Part model, mm, in its own coordinate system. Give positions to 0.01 mm unless a question says otherwise; leave off trailing zeros. Write each loop counter-clockwise with the first axis right and the second up, starting at its lowest first coordinate (ties: lowest second). Pieces come first, ordered by that corner, then holes. Notation, with made-up numbers: (48, 65.5) - (102, 65.5) arc R19 cw to (102, 69.5) - close; hole circle Ø10 at (76.5, 8). An arc over 180 degrees is marked (long way). Answer in a Markdown table with one row per item. Add a question column.
1. Probe line 1 along X through (y, z) = (3.5, -6.5); line 2 along X through (y, z) = (4.75, -0.25); line 3 along X through (y, z) = (6.75, 4). List the from-to ranges inside material, lowest first.
2. Band-saw the part on A-A on y = 6.5. Write the cut outline in (x, z), plus the area to 3 significant figures.
3. Drop flat-ended pins along their axis: pin 1 Ø2 at (y, z) = (7, 6) entering from -X; pin 2 Ø11 at (x, z) = (0, 0) entering from -Y; pin 3 Ø2 at (y, z) = (5.5, 2.5) entering from -X. Give the stop position or say it passes through.
4. Pull direction Z, two halves, no side cores. Call faces 1 (the conical face through (-6.77, 7.72, 11.66)), 2 (the flat face through (-11.2, 3.9, -6.6)), 3 (the cylindrical face through (1.802, 4.056, 5.723)): released by +Z, released by -Z, zero draft, split by the parting line, or undercut.
5. Band-saw the part on B-B on y = 0.5. Write the cut outline in (x, z).
```python
from build123d import *

# Parameters (mm, degrees)
BOSS_EXTRUDE1_DEPTH     = 8
SKETCH2_R               = 6
CUT_EXTRUDE1_DEPTH      = 22.408720964
SKETCH3_OUTSIDE_W       = 67.838
SKETCH3_OUTSIDE_H       = 63.816
SKETCH3_OUTSIDE_R       = 13
CUT_EXTRUDE2_DEPTH      = 8
CUT_EXTRUDE2_DRAFT      = -60
MIRROR1_COPY_1_SKETCH_W = 67.838
MIRROR1_COPY_1_SKETCH_H = 63.816
MIRROR1_COPY_1_SKETCH_R = 13
MIRROR1_COPY_1_DEPTH    = 8
MIRROR1_COPY_1_DRAFT    = -60


with BuildPart() as part:
    # Sketch1 → Boss-Extrude1 (new body)
    with BuildSketch(Plane(origin=(0, 0, 0), x_dir=(1, 0, 0), z_dir=(0, 1, 0))):
        Polygon((7.505553499, -13), (15.011106999, 0), (7.505553499, 13), (-7.505553499, 13), (-15.011106999, 0), (-7.505553499, -13), align=None)
    extrude(amount=BOSS_EXTRUDE1_DEPTH)

    # Sketch2 → Cut-Extrude1 (cut, through all)
    with BuildSketch(Plane(origin=(0, 8, 0), x_dir=(1, 0, 0), z_dir=(0, 1, 0))):
        with Locations(Location((0, 0, 0), (0, 0, 270))):
            Circle(SKETCH2_R)
    extrude(amount=-CUT_EXTRUDE1_DEPTH, mode=Mode.SUBTRACT)


with BuildPart() as cut_extrude2_tool:
    # Sketch3 outside → Cut-Extrude2 (with draft: the straight prism first)
    with BuildSketch(Plane(origin=(0, 8, 0), x_dir=(1, 0, 0), z_dir=(0, 1, 0))):
        Rectangle(SKETCH3_OUTSIDE_W, SKETCH3_OUTSIDE_H)
        Circle(SKETCH3_OUTSIDE_R, mode=Mode.SUBTRACT)
    extrude(amount=-CUT_EXTRUDE2_DEPTH)
    # Cut-Extrude2: the draft: its side faces are tilted about the plane it starts from
    cut_extrude2_sides = [cut_extrude2_tool.faces().sort_by_distance(p)[0] for p in [
        (0, 4, 31.908),
        (33.919, 4, 0),
        (0, 4, -31.908),
        (-33.919, 4, 0),
        (-13, 4, 0),
    ]]
    draft(cut_extrude2_sides, Plane(origin=(0, 8, 0), x_dir=(1, 0, 0), z_dir=(0, 1, 0)), CUT_EXTRUDE2_DRAFT)


with BuildPart() as part_1:
    add(part.part)

    # Cut-Extrude2: cut by cut_extrude2_tool
    add(cut_extrude2_tool.part, mode=Mode.SUBTRACT)


with BuildPart() as mirror1_copy_1_tool:
    # Mirror1 copy 1 sketch → Mirror1 copy 1 (with draft: the straight prism first)
    with BuildSketch(Plane.XZ):
        Rectangle(MIRROR1_COPY_1_SKETCH_W, MIRROR1_COPY_1_SKETCH_H)
        Circle(MIRROR1_COPY_1_SKETCH_R, mode=Mode.SUBTRACT)
    extrude(amount=-MIRROR1_COPY_1_DEPTH)
    # Mirror1 copy 1: the draft: its side faces are tilted about the plane it starts from
    mirror1_copy_1_sides = [mirror1_copy_1_tool.faces().sort_by_distance(p)[0] for p in [
        (0, 4, 31.908),
        (33.919, 4, 0),
        (0, 4, -31.908),
        (-33.919, 4, 0),
        (-13, 4, 0),
    ]]
    draft(mirror1_copy_1_sides, Plane.XZ, MIRROR1_COPY_1_DRAFT)


with BuildPart() as part_2:
    add(part_1.part)

    # Mirror1 copy 1: cut by mirror1_copy_1_tool
    add(mirror1_copy_1_tool.part, mode=Mode.SUBTRACT)


solid = part_2.part
```
Values:
| question | item | result |
|---|---|---|
| 1 | line 1 | x = -11.26 to 11.26 |
| 1 | line 2 | x = -14.87 to -5.99, 5.99 to 14.87 |
| 1 | line 3 | x = -12.7 to -4.47, 4.47 to 12.7 |
| 2 | outline | (-15.01, 0) - (-7.51, -13) - (7.51, -13) - (15.01, 0) - (7.51, 13) - (-7.51, 13) - close; hole circle Ø12 at (0, 0) |
| 2 | area | 472 mm² |
| 3 | pin 1 | stops at x = -12.12 |
| 3 | pin 2 | passes through |
| 3 | pin 3 | stops at x = -14.15 |
| 4 | face 1 | released by +Z |
| 4 | face 2 | released by -Z |
| 4 | face 3 | undercut |
| 5 | outline | (-13.67, -2.32) - (-8.85, -10.68) arc R13.87 ccw to (-4.82, -13) - (4.82, -13) arc R13.87 ccw to (8.85, -10.68) - (13.67, -2.32) arc R13.87 ccw to (13.67, 2.32) - (8.85, 10.68) arc R13.87 ccw to (4.82, 13) - (-4.82, 13) arc R13.87 ccw to (-8.85, 10.68) - (-13.67, 2.32) arc R13.87 ccw to start; hole circle Ø12 at (0, 0) |
